from build123d import *

# Parameters (mm, degrees)
BOSS_EXTRU_1_DEPTH          = 20
ENL_V_MAT_EXTRU_1_REACH     = 77.705
ESQUISSE2_R                 = 1.5
D_GAGEMENT_M31_D            = 3.4
D_GAGEMENT_M31_DEPTH        = 57.5
D_GAGEMENT_M31_TIP          = 1.021463052
CONG_1_R                    = 10
CONG_2_R                    = 5
ENL_V_START                 = 0.83484861
ENL_V_MAT_EXTRU_2_OUTLINE_W = 4
ENL_V_MAT_EXTRU_2_OUTLINE_H = 5
ENL_V_MAT_EXTRU_2_DEPTH     = 3.16515139


# Read off the part's stored shape, not the designer's step: Enlèv. mat.-Extru.2
with BuildPart() as part:
    # Esquisse1 → Boss.-Extru.1 (new body)
    with BuildSketch(Plane.XY):
        Polygon((0, 0), (4, 0), (4, 41), (53.5, 41), (53.5, 0), (57.5, 0), (57.5, 45), (0, 45), align=None)
    extrude(amount=BOSS_EXTRU_1_DEPTH)

    # Enlèv. mat.-Extru.1: up to this face of the body (flat: up to its plane)
    enl_v_mat_extru_1_end = Plane(part.part.faces().sort_by_distance((0, 22.5, 10))[0])
    # Esquisse2 → Enlèv. mat.-Extru.1 (cut, up to the picked face)
    with BuildSketch(Plane(origin=(57.5, 0, 0), x_dir=(0, 0, -1), z_dir=(1, 0, 0)), mode=Mode.PRIVATE) as enl_v_mat_extru_1_sk1:
        with Locations((-10, 5.5)):
            Circle(ESQUISSE2_R)
    enl_v_mat_extru_1_tool1 = split(extrude(enl_v_mat_extru_1_sk1.sketch, amount=-ENL_V_MAT_EXTRU_1_REACH, mode=Mode.PRIVATE), bisect_by=enl_v_mat_extru_1_end, keep=Keep.BOTH, mode=Mode.PRIVATE)
    add(enl_v_mat_extru_1_tool1.solids().sort_by(Axis((57.5, 5.5, 10), (-1, 0, 0)))[0], mode=Mode.SUBTRACT)

    # Dégagement M31
    with Locations(Plane(origin=(57.5, 0, 0), x_dir=(0, 0, -1), z_dir=(1, 0, 0))):
        with Locations((-10, 5.5)):
            Hole(D_GAGEMENT_M31_D / 2, depth=D_GAGEMENT_M31_DEPTH)
            with Locations((0, 0, -(D_GAGEMENT_M31_DEPTH + D_GAGEMENT_M31_TIP / 2))):  # 118° drill point
                Cone(0, D_GAGEMENT_M31_D / 2, D_GAGEMENT_M31_TIP, mode=Mode.SUBTRACT)

    # Congé1
    cong_1_edges = [part.edges().sort_by_distance(p)[0] for p in [
        (55.5, 0, 0),
        (55.5, 0, 20),
        (2, 0, 0),
        (2, 0, 20),
    ]]
    fillet(cong_1_edges, radius=CONG_1_R - 0.0001)  # a hair under: the kernel refuses the full size

    # Congé2
    cong_2_edges = [part.edges().sort_by_distance(p)[0] for p in [
        (0, 45, 10),
        (57.5, 45, 10),
    ]]
    fillet(cong_2_edges, radius=CONG_2_R)

    # Enlèv. mat.-Extru.2 outline → Enlèv. mat.-Extru.2 (cut)
    with BuildSketch(Plane(origin=(0, 0, 0), x_dir=(1, 0, 0), z_dir=(0, 1, 0)).offset(ENL_V_START)):
        with Locations((2, -3.5)):
            Rectangle(ENL_V_MAT_EXTRU_2_OUTLINE_W, ENL_V_MAT_EXTRU_2_OUTLINE_H)
    extrude(amount=ENL_V_MAT_EXTRU_2_DEPTH, mode=Mode.SUBTRACT)


solid = part.part
The model under review builds one solid part; all positions refer to its coordinate system, in mm. A direction names the side the tool comes from. Give positions to 0.01 mm unless a question says otherwise; leave off trailing zeros. Write each loop counter-clockwise with the first axis right and the second up, starting at its lowest first coordinate (ties: lowest second). Pieces come first, ordered by that corner, then holes.
1. For P1, Ø10, axis at x = 23.5, z = 12, coming from the -Y side; P2, Ø2.5, axis at y = 5.5, z = 10, coming from the +X side; P3, Ø2.5, axis at x = 1, y = 2.5, coming from the -Z side; P4, Ø4, axis at y = 5.5, z = 10, coming from the +X side, all flat-tipped, find the tip position at first contact; note any pin that passes through.
2. Wall thickness on L1, parallel to X at y = 8.5, z = 17.5; L2, parallel to Y at x = 8, z = 2; L3, parallel to Y at x = 56.45, z = 10: over which ranges is each line inside the solid? List them lowest first.
3. Tool access review of faces 5 (the flat face through (2, 4, 4)), 6 (the flat face through (4, 20, 10)), 7 (the cylindrical face through (55.53, 2.85, 3.01)): name each direction out of +Z, -Z, +X, -X, +Y, -Y from which nothing blocks a thin tool from reaching the whole face with its end or side.
4. Draft analysis for pull direction X (two halves, no side actions). For faces 1 (the flat face through (28, 41, 10)), 2 (the flat face through (53.5, 21, 10)), 3 (the flat face through (57.5, 20, 10)), 4 (the cylindrical face through (1.97, 3.84, 9.63)), state which applies: +X half, -X half, draft (parallel to the pull), parting line (faces both ways), or undercut.
5. Add section B-B, the plane y = 5.5. Write out the cut boundary in (x, z), plus the area to 3 significant figures.
6. Add section A-A, the plane y = 26. Write out the cut boundary in (x, z), plus the area to 3 significant figures.
7. Add section D-D, the plane z = 7.25. Write out the cut boundary in (x, y), plus the area to 3 significant figures.
8. Add section C-C, the plane x = 37.5. Write out the cut boundary in (y, z), plus the area to 3 significant figures.
Worked answers:
1. P1: stops at y = 41
1. P2: passes through
1. P3: stops at z = 6
1. P4: stops at x = 57.5
2. L1: x = 0 to 4, 53.5 to 57.5
2. L2: y = 41 to 45
2. L3: y = 0 to 3.8, 7.2 to 43.07
3. face 5: -Z, -X, -Y
3. face 6: +Z, -Z, -Y
3. face 7: -Z, +X, -X, -Y
4. face 1: undercut
4. face 2: undercut
4. face 3: +X half
4. face 4: draft
5. outline: (0, 1.07) - (4, 1.07) - (4, 8.3) - (0, 8.3) - close; (0, 11.7) - (4, 11.7) - (4, 18.93) - (0, 18.93) - close; (53.5, 1.07) - (57.5, 1.07) - (57.5, 8.3) - (53.5, 8.3) - close; (53.5, 11.7) - (57.5, 11.7) - (57.5, 18.93) - (53.5, 18.93) - close
5. area: 116 mm2
6. outline: (0, 0) - (4, 0) - (4, 20) - (0, 20) - close; (53.5, 0) - (57.5, 0) - (57.5, 20) - (53.5, 20) - close
6. area: 160 mm2
7. outline: (0, 0.39) - (4, 0.39) - (4, 41) - (53.5, 41) - (53.5, 0.39) - (57.5, 0.39) - (57.5, 40) arc R5 ccw to (52.5, 45) - (5, 45) arc R5 ccw to (0, 40) - close
7. area: 544 mm2
8. outline: (41, 0) - (45, 0) - (45, 20) - (41, 20) - close
8. area: 80.0 mm2
